Design review of the part shown in the three views and the two pictorial views. Dimensions are in mm from the part's minimum x, y and z. A direction names the side the tool comes from. Coordinates: 2 decimals unless noted, no trailing zeros. Loops run counter-clockwise (first coordinate to the right, second up) from the corner with the lowest first, then second, coordinate; pieces in that order, holes last. Notation, with made-up numbers: M 65.5,87.25 L 118.5,87.25 A16 cw 118.5,105.25 Z; hole C 53,16.25 d10. An arc over 180 degrees is marked long. Use CSV: the item, a comma, the result in double quotes. Start each with the question number.
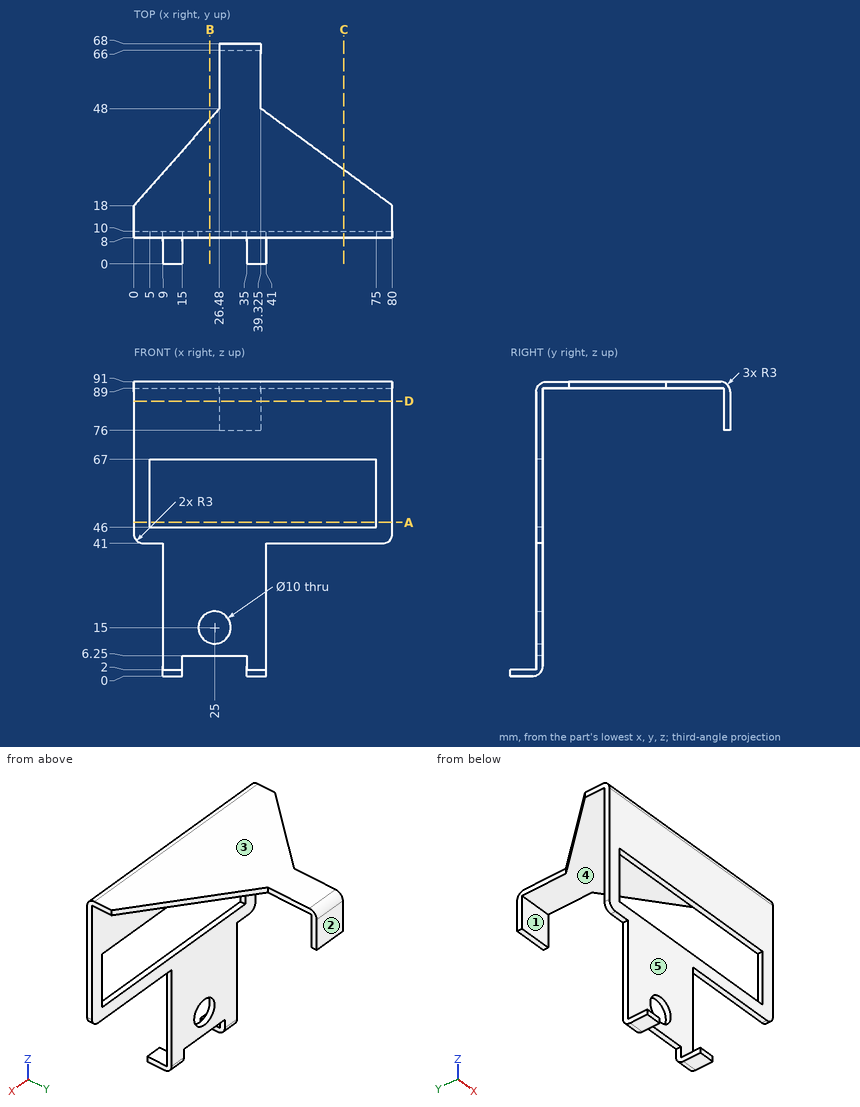
1. Add section D-D (z = 85). Write out the cut boundary in (x, y) (1 decimal).
2. Add section A-A (z = 47.5). Write out the cut boundary in (x, y).
3. Insertion check: pin 1 Ø0.6 at (x, y) = (54, 9) entering from -Z; pin 2 Ø6 at (x, y) = (10, 30.5) entering from -Z; pin 3 Ø3 at (y, z) = (6, 25.5) entering from -X; pin 4 Ø1.9 at (y, z) = (4, 2.5) entering from +X. Each pin has a flat end and moves straight along its axis. Give the tip position at first contact, or say it passes through.
4. Draft analysis for pull direction Y (two halves, no side actions). For the marked faces 1, 2 and 3, state which applies: released by +Y, released by -Y, zero draft, split by the parting line, or undercut.
5. To check wall thickness, follow line 1 along Z through (x, y) = (25, 8.6); line 2 along Z through (x, y) = (25, 9.05); line 3 along Y through (x, z) = (15, 19.5). State the ranges of each line that lie inside material, in increasing order.
6. Add section B-B (x = 23.5). Write out the cut boundary in (y, z).
7. Add section C-C (x = 65). Write out the cut boundary in (y, z).
8. For the marked faces 4 and 5, list the 3-axis set-ups (+Z, -Z, +X, -X, +Y, -Y) from which the entire face can be reached by the end or side of a thin tool; tool diameter is ignored.
Solved:
1,outline,"M 0,8 L 80,8 L 80,10 L 0,10 Z; M 26.5,66 L 39.3,66 L 39.3,68 L 26.5,68 Z"
2,outline,"M 0,8 L 5,8 L 5,10 L 0,10 Z; M 75,8 L 80,8 L 80,10 L 75,10 Z"
3,pin 1,"stops at z = 41"
3,pin 2,"stops at z = 89"
3,pin 3,"passes through"
3,pin 4,"stops at x = 41"
4,face 1,"undercut"
4,face 2,"released by +Y"
4,face 3,"zero draft"
5,line 1,"z = 6.25 to 10, 20 to 46, 67 to 89.8"
5,line 2,"z = 6.25 to 10, 20 to 46, 67 to 90.28"
5,line 3,"y = 8 to 10"
6,outline,"M 8,6.25 L 10,6.25 L 10,10.23 L 8,10.23 Z; M 8,19.77 L 10,19.77 L 10,46 L 8,46 Z; M 8,67 L 10,67 L 10,89 L 44.62,89 L 44.62,91 L 11,91 A3 ccw 8,88 Z"
7,outline,"M 8,41 L 10,41 L 10,46 L 8,46 Z; M 8,67 L 10,67 L 10,89 L 29.06,89 L 29.06,91 L 11,91 A3 ccw 8,88 Z"
8,face 4,"-Z, +X, -X"
8,face 5,"+Z, +X, -X, -Y"
